from build123d import *

# Parameters (mm, degrees)
BOX002_W          = 80
BOX002_H          = 100
BOX002_DEPTH      = 10
BOX_W             = 10
BOX_H             = 10
BOX_DEPTH         = 10.8
CYLINDER002_R     = 2.15
CYLINDER002_DEPTH = 10.8
CYLINDER_R        = 22.75
CYLINDER_DEPTH    = 60
CYLINDER001_R     = 27.75
CYLINDER001_DEPTH = 15
SKETCH025_R       = 48.85367
POCKET023_DEPTH   = 4
SKETCH026_R       = 13.5
POCKET024_DEPTH   = 5.5
SKETCH027_R       = 4
POCKET025_DEPTH   = 20
SKETCH028_R       = 1.7
POCKET026_DEPTH   = 56.001
SKETCH029_R       = 3.4
POCKET027_DEPTH   = 40
POCKET028_DEPTH   = 19
SKETCH050_R       = 33.40384
SKETCH050_R_2     = 22.65
POCKET041_DEPTH   = 45


with BuildPart() as cutcube001:
    # Box002 → Box002 (new body)
    with BuildSketch(Plane(origin=(-40, -0.5, -1), x_dir=(1, 0, 0), z_dir=(0, 0, 1))):
        with Locations((40, 50)):
            Rectangle(BOX002_W, BOX002_H)
    extrude(amount=BOX002_DEPTH)


with BuildPart() as cube:
    # Box → Box (new body)
    with BuildSketch(Plane(origin=(-5, 1.536842, 0), x_dir=(1, 0, 0), z_dir=(0, 0, 1))):
        with Locations((5, 5)):
            Rectangle(BOX_W, BOX_H)
    extrude(amount=BOX_DEPTH)


with BuildPart() as motor_shaft_hole:
    # Cylinder002 → Cylinder002 (new body)
    with BuildSketch(Plane.XY):
        Circle(CYLINDER002_R)
    extrude(amount=CYLINDER002_DEPTH)

    # Cut: cut Cube
    add(cube.part, mode=Mode.SUBTRACT)


with BuildPart() as motor_shaft_hole_1:
    # Cut placement: moved
    add(motor_shaft_hole.part.moved(Location((0, 0, 49.2))))


with BuildPart() as cylinder_plug_inner:
    # Cylinder → Cylinder (new body)
    with BuildSketch(Plane.XY):
        Circle(CYLINDER_R)
    extrude(amount=CYLINDER_DEPTH)


with BuildPart() as body002:
    # Cylinder001 → Cylinder001 (new body)
    with BuildSketch(Plane.XY.offset(45)):
        Circle(CYLINDER001_R)
    extrude(amount=CYLINDER001_DEPTH)

    # Fusion: union Cylinder_plug_inner
    add(cylinder_plug_inner.part)

    # Cut001: cut Motor_shaft_hole
    add(motor_shaft_hole_1.part, mode=Mode.SUBTRACT)

    # Cut003: cut CutCube001
    add(cutcube001.part, mode=Mode.SUBTRACT)


with BuildPart() as body002_1:
    # Cut003 placement: moved
    add(body002.part.moved(Location((135, 0, 0))))


with BuildPart() as body002_2:
    # BaseFeature001 placement: moved
    add(body002_1.part.moved(Location((-135, 0, 0))))

    # Sketch025 (on Face5 of BaseFeature001) → Pocket023 (cut)
    with BuildSketch(Plane.XY.offset(60)):
        Circle(SKETCH025_R)
    extrude(amount=-POCKET023_DEPTH, mode=Mode.SUBTRACT)

    # Sketch026 (on Face3 of Pocket023) → Pocket024 (cut)
    with BuildSketch(Plane.XY.offset(56)):
        Circle(SKETCH026_R)
    extrude(amount=-POCKET024_DEPTH, mode=Mode.SUBTRACT)

    # Sketch027 (on Face3 of Pocket024) → Pocket025 (cut)
    with BuildSketch(Plane.XY.offset(56)):
        Circle(SKETCH027_R)
    extrude(amount=-POCKET025_DEPTH, mode=Mode.SUBTRACT)

    # Sketch028 (on Face3 of Pocket025) → Pocket026 (cut, through all)
    with BuildSketch(Plane.XY.offset(56)):
        with Locations((-4.75, 8.25)):
            Circle(SKETCH028_R)
        with Locations((4.75, 8.25)):
            Circle(SKETCH028_R)
        with Locations((4.75, -8.25)):
            Circle(SKETCH028_R)
        with Locations((-4.75, -8.25)):
            Circle(SKETCH028_R)
        with Locations((-9.5, 0)):
            Circle(SKETCH028_R)
        with Locations((9.5, 0)):
            Circle(SKETCH028_R)
    extrude(amount=-POCKET026_DEPTH, mode=Mode.SUBTRACT)

    # Sketch029 (on Face6 of Pocket026) → Pocket027 (cut)
    with BuildSketch(Plane(origin=(0, 0, 0), x_dir=(1, 0, 0), z_dir=(0, 0, -1))):
        with Locations((-4.75, 8.25)):
            Circle(SKETCH029_R)
        with Locations((4.75, 8.25)):
            Circle(SKETCH029_R)
        with Locations((9.5, 0)):
            Circle(SKETCH029_R)
        with Locations((-9.5, 0)):
            Circle(SKETCH029_R)
        with Locations((-4.75, -8.25)):
            Circle(SKETCH029_R)
        with Locations((4.75, -8.25)):
            Circle(SKETCH029_R)
    extrude(amount=-POCKET027_DEPTH, mode=Mode.SUBTRACT)

    # Sketch030 (on DatumPlane) → Pocket028 (cut)
    with BuildSketch(Plane.XZ.offset(-28)):
        with BuildLine():
            ThreePointArc((-2.723427, 53.237899), (0, 50.514472), (2.723427, 53.237899))
            Line((2.723427, 53.237899), (2.723427, 64.839276))
            ThreePointArc((2.723427, 64.839276), (0, 67.562703), (-2.723427, 64.839276))
            Line((-2.723427, 64.839276), (-2.723427, 53.237899))
        make_face()
    extrude(amount=POCKET028_DEPTH, mode=Mode.SUBTRACT)

    # Sketch050 (on Face10 of Pocket028) → Pocket041 (cut)
    with BuildSketch(Plane(origin=(0, 0, 0), x_dir=(1, 0, 0), z_dir=(0, 0, -1))):
        Circle(SKETCH050_R)
        Circle(SKETCH050_R_2, mode=Mode.SUBTRACT)
    extrude(amount=-POCKET041_DEPTH, mode=Mode.SUBTRACT)


with BuildPart() as body002_3:
    # Body002 placement: moved
    add(body002_2.part.moved(Location((0, 0, -67))))


solid = body002_3.part
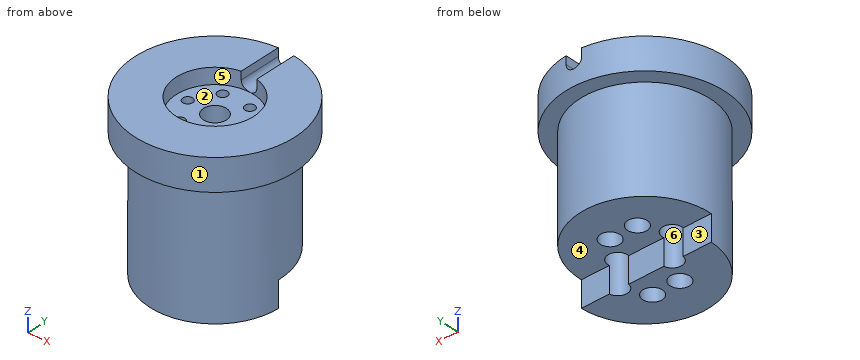
Build history of the part. All positions in model axes, mm. Face numbers are marked on the shaded views. A direction names the side the tool comes from. Coordinates: 2 decimals unless noted, no trailing zeros. Order: outer loops, then holes, each group sorted by start corner. A loop starts at its lowest first (then second) coordinate and runs counter-clockwise, first axis right, second up. Notation, with made-up numbers: (23.5, -36.75) - (37.5, -36.75) arc R25 cw to (37.5, -6.75) - close; hole circle Ø5 at (62, 32). An arc over 180 degrees is marked (long way). Write each question's results on one line, items separated by ' | '. Start each with the question number.
Item 1: Wall check: probe 1 along X at (y, z) = (0, -48); probe 2 along Y at (x, z) = (0, -28); probe 3 along Y at (x, z) = (-4, -46). Give the ranges that are in metal, low to high. Write a range as [from, to].
Item 2: Band-saw the part on A-A on z = -25. Write the cut outline in (x, y).
Item 3: Band-saw the part on B-B on y = 8.25. Write the cut outline in (x, z), and give its area (3 significant figures).
Item 4: Tool access for the marked faces 4, 5 and 6: list every direction of +Z, -Z, +X, -X, +Y, -Y with a clear straight run to the whole face (end or side of a thin tool).
Item 5: Band-saw the part on D-D on x = -9.5. Write the cut outline in (y, z).
Item 6: Flat gauge pins, fed straight in: pin 1 (1.5 mm diameter, centred on y = 1.5, z = -26.5, fed in from +X); pin 2 (1.5 mm diameter, centred on y = 5.5, z = -45.5, fed in from -X); pin 3 (5.5 mm diameter, centred on x = -4.75, y = -8.25, fed in from -Z); pin 4 (16 mm diameter, centred on x = 0, y = 0, fed in from -Z). Where does each tip first touch, or does it go through?
Item 7: Band-saw the part on C-C on z = -33. Write the cut outline in (x, y).
Item 8: Mould opens along Y. For the marked faces 1, 2 and 3 say: released by +Y, released by -Y, zero draft, split by the parting line, or undercut.
Numbers:
1) probe 1: [-22.65, -12.9], [-6.1, 6.1], [12.9, 22.65] | probe 2: [-22.65, -4], [4, 22.65] | probe 3: [-22.29, -11.57], [-4.93, 4.93], [11.57, 22.29]
2) outline: circle Ø45.3 at (0, 0); hole circle Ø3.4 at (-9.5, 0); hole circle Ø3.4 at (-4.75, -8.25); hole circle Ø3.4 at (-4.75, 8.25); hole circle Ø8 at (0, 0); hole circle Ø3.4 at (4.75, -8.25); hole circle Ø3.4 at (4.75, 8.25); hole circle Ø3.4 at (9.5, 0)
3) outline: (-26.5, -22) - (-21.09, -22) - (-21.09, -58) - (-8.15, -58) - (-8.15, -27) - (-6.45, -27) - (-6.45, -16.5) - (-10.69, -16.5) - (-10.69, -11) - (-26.5, -11) - close; (-3.05, -27) - (-1.35, -27) - (-1.35, -58) - (1.35, -58) - (1.35, -27) - (3.05, -27) - (3.05, -16.5) - (-3.05, -16.5) - close; (6.45, -27) - (8.15, -27) - (8.15, -58) - (21.09, -58) - (21.09, -22) - (26.5, -22) - (26.5, -11) - (10.69, -11) - (10.69, -16.5) - (6.45, -16.5) - close | area: 1,490 mm^2
4) face 4: -Z, +X, -X, +Y | face 5: +Z | face 6: -Z
5) outline: (-26.07, -22) - (-20.56, -22) - (-20.56, -67) - (-3.4, -67) - (-3.4, -27) - (-1.7, -27) - (-1.7, -16.5) - (-9.59, -16.5) - (-9.59, -11) - (-26.07, -11) - close; (1.7, -27) - (3.4, -27) - (3.4, -58) - (20.56, -58) - (20.56, -22) - (26.07, -22) - (26.07, -11) - (9.59, -11) - (9.59, -16.5) - (1.7, -16.5) - close
6) pin 1: x = 22.64 | pin 2: x = -22.15 | pin 3: z = -27 | pin 4: z = -67
7) outline: circle Ø45.3 at (0, 0); hole circle Ø6.8 at (-9.5, 0); hole circle Ø6.8 at (-4.75, -8.25); hole circle Ø6.8 at (-4.75, 8.25); hole circle Ø6.8 at (4.75, -8.25); hole circle Ø6.8 at (4.75, 8.25); hole circle Ø6.8 at (9.5, 0)
8) face 1: split by the parting line | face 2: undercut | face 3: released by +Y
